Can you work these out from the model? Positions are in its coordinate system, mm. A direction names the side the tool comes from. Round coordinates to 2 decimals unless told otherwise and drop trailing zeros. Loops run counter-clockwise (first coordinate to the right, second up) from the corner with the lowest first, then second, coordinate; pieces in that order, holes last.
Autodesk Inventor part; units mm, degrees
ref_plane "YZ Plane" through (0, 0, 0) normal (1, 0, 0) x (0, 1, 0)
ref_plane "XZ Plane" through (0, 0, 0) normal (0, 1, 0) x (-1, 0, 0)
ref_plane "XY Plane" through (0, 0, 0) normal (0, 0, 1) x (1, 0, 0)
sketch "Эскиз1" plane through (0, 0, 0) normal (0, 0, 1) x (1, 0, 0)
  arc A0 (3.75, 0) -> (-3.75, 0) centre (0, 0) ccw
  line L0 (-3.75, 0) -> (-13.75, 0) construction
  line L1 (-13.75, 4.8279) -> (13.75, 4.8279)
  line L2 (-13.75, 0) -> (-3.75, 0)
  line L3 (3.75, 0) -> (13.75, 0)
  line L4 (0, 9.2451) -> (0, -5.452)
  line L5 (-13.75, 0) -> (-13.75, 4.8279)
  line L6 (13.75, 0) -> (13.75, 4.8279)
  point P0 (0, 4.8279)
  dimension "d25" = 3.75
extrude "Выдавливание1" add sketch "Эскиз1" along normal blind 30
sketch "Эскиз4" plane through (0, 0, 30) normal (0, 0, 1) x (1, 0, 0)
  circle A0 centre (0, 0) radius 4.25
  dimension "d22" = 8.5
extrude "Выдавливание4" cut sketch "Эскиз4" against normal blind 3
sketch "Эскиз5" plane through (-13.75, 0, 0) normal (0, -1, 0) x (1, 0, 0)
  line L0 (23.75, -2.1369) -> (23.75, 32.4902)
  line L1 (27.5, 30) -> (0, 30)
  line L2 (0, 30) -> (3.5, 30)
  line L3 (0, 30) -> (0, 0)
  line L4 (0, 0) -> (27.5, 0)
  line L5 (0, 0) -> (27.5, 0)
  line L6 (27.5, 0) -> (27.5, 30)
  line L7 (27.5, 30) -> (24, 30)
  line L8 (3.5, 4) -> (24, 4)
  line L9 (24, 4) -> (24, 30)
  line L10 (3.5, 30) -> (3.5, 4)
  point P0 (13.75, 0)
  dimension "d26" = 3.5
  dimension "d27" = 3.5
extrude "Выдавливание5" add sketch "Эскиз5" along normal blind 25 contours L4 L3 L1 L10 L8 L0 | L0 L8 L9 L1 L6 L4
sketch "Эскиз6" plane through (-3.75, 0, 4) normal (0, 0, 1) x (1, 0, 0)
  circle A0 centre (3.75, 0) radius 3.75
extrude "Выдавливание6" cut sketch "Эскиз6" against normal blind 25
properties part number "mini_holder"
(1) If we section it at A-A, the plane x = 0: List the corners of the cut face in (y, z) for me, then the cut area to 3 significant figures.
Worked answers:
outline: (-25, 0) - (-3.75, 0) - (-3.75, 4) - (-25, 4) - close; (3.75, 0) - (4.83, 0) - (4.83, 30) - (4.25, 30) - (4.25, 27) - (3.75, 27) - close
area: 116 mm2
(2) If we section it at C-C, the plane y = -10.5: List the corners of the cut face in (x, z) for me.
Worked answers:
outline: (-13.75, 0) - (13.75, 0) - (13.75, 30) - (10.25, 30) - (10.25, 4) - (-10.25, 4) - (-10.25, 30) - (-13.75, 30) - close
(3) If we section it at B-B, the plane z = 2.75: List the corners of the cut face in (x, y) for me, then the cut area to 3 significant figures.
Worked answers:
outline: (-13.75, -25) - (13.75, -25) - (13.75, 4.83) - (-13.75, 4.83) - close; hole circle Ø7.5 at (0, 0)
area: 776 mm2
(4) Will these pins go through, and if not, where does the flat tip stop? P1, Ø3, axis at x = 3, y = -9, coming from the +Z side; P2, Ø3, axis at x = -7.5, z = 14, coming from the -Y side.
Worked answers:
P1: stops at z = 4
P2: stops at y = 0
(5) If I drill on line 1 (X direction, y = -2.5, z = 24); line 2 (Y direction, x = 0, z = 15.75); line 3 (Z direction, x = -9.5, y = -5.5), over which ranges is the centre line in solid material (lowest first)?
Worked answers:
line 1: x = -13.75 to -10.25, 10.25 to 13.75
line 2: y = 3.75 to 4.83
line 3: z = 0 to 4
(6) If we mould it in two halves opening along X, with no side actions, what happens to faces 1 (the flat face through (-13.75, -10, 15)), 2 (the flat face through (0, -12, 4)), 3 (the flat face through (13.75, -10, 15))? For each: released by +X, released by -X, zero draft, split by the parting line, or undercut.
Worked answers:
face 1: released by -X
face 2: undercut
face 3: released by +X
(7) For faces 4 (the flat face through (-10.25, -12, 17)), 5 (the cylindrical face through (-0.81, 3.66, 13.31)), which set-ups out of +Z, -Z, +X, -X, +Y, -Y let a thin tool reach every point of the face, with its end or its side?
Worked answers:
face 4: +Z, -Y
face 5: +Z, -Z
(8) If we section it at D-D, the plane x = -5.5: List the corners of the cut face in (y, z) for me.
Worked answers:
outline: (-25, 0) - (4.83, 0) - (4.83, 30) - (0, 30) - (0, 4) - (-25, 4) - close
